```python
from build123d import *

# Parameters (mm, degrees)
F0_R     = 12.7
F1_DEPTH = 60.325
F2_W     = 51.3197111964
F2_H     = 22.6086642011
F3_DEPTH = 55.88
F4_DEPTH = 19.05
F5_DEPTH = 19.05
F6_R     = 6.35
F7_DEPTH = 22.353


with BuildPart() as f1:
    # F0 (on Front) → F1 (new body)
    with BuildSketch(Plane.XZ):
        with BuildLine():
            ThreePointArc((-47.1229317725, 0), (-49.3023607466, 0.8214167326), (-50.3974654162, 2.876990099))
            ThreePointArc((-50.3974654162, 2.876990099), (-89.3551798917, 14.7530576713), (-72.5635393124, -22.352))
            Line((-72.5635393124, -22.352), (19.2828606876, -22.352))
            Line((19.2828606876, -22.352), (13.2884606876, 0))
            Line((13.2884606876, 0), (-47.1229317725, 0))
        make_face()
        with Locations((-72.5635393124, 0)):
            Circle(F0_R, mode=Mode.SUBTRACT)
        Polygon((13.2884606876, 0), (19.2828606876, -22.352), (44.6828606876, -22.352), (44.6828606876, 0), align=None)
        with BuildLine():
            Line((44.6828606876, 0), (44.6828606876, -22.352))
            Line((44.6828606876, -22.352), (121.6448606876, -22.352))
            Line((121.6448606876, -22.352), (121.6448606876, -7.874))
            ThreePointArc((121.6448606876, -7.874), (119.3386194827, -2.3062412049), (113.7708606876, 0))
            Line((113.7708606876, 0), (80.8270606876, 0))
            Line((80.8270606876, 0), (44.6828606876, 0))
        make_face()
    extrude(amount=-F1_DEPTH)

    # F2 (on Top) → F3 (cut, symmetric)
    with BuildSketch(Plane.XY):
        with Locations((-69.2556837142, 30.3035321005)):
            Rectangle(F2_W, F2_H)
    extrude(amount=F3_DEPTH, both=True, mode=Mode.SUBTRACT)

    # F0 (on Front) → F4 (cut)
    with BuildSketch(Plane.XZ):
        Polygon((13.2884606876, 0), (19.2828606876, -22.352), (44.6828606876, -22.352), (44.6828606876, 0), align=None)
    extrude(amount=-F4_DEPTH, mode=Mode.SUBTRACT)

    # F0 (on Front) → F5 (join)
    with BuildSketch(Plane.XZ):
        with BuildLine():
            ThreePointArc((58.4750606876, 34.798), (54.9008760492, 16.0823576341), (44.6828606876, 0))
            Line((44.6828606876, 0), (80.8270606876, 0))
            ThreePointArc((80.8270606876, 0), (78.4921940962, 0.9671334085), (77.5250606876, 3.302))
            Line((77.5250606876, 3.302), (77.5250606876, 29.718))
            ThreePointArc((77.5250606876, 29.718), (76.0371631361, 33.3101024484), (72.4450606876, 34.798))
            Line((72.4450606876, 34.798), (58.4750606876, 34.798))
        make_face()
    extrude(amount=-F5_DEPTH)

    # F6 (on Top) → F7 (cut, through all)
    with BuildSketch(Plane.XY):
        with Locations((82.7828606876, 37.973)):
            Circle(F6_R)
    extrude(amount=-F7_DEPTH, mode=Mode.SUBTRACT)


solid = f1.part
```
Geometry check sheet. Reference: the model listing, model coordinates, mm. A direction names the side the tool comes from. Coordinates: 2 decimals unless noted, no trailing zeros. Order: outer loops, then holes, each group sorted by start corner. A loop starts at its lowest first (then second) coordinate and runs counter-clockwise, first axis right, second up.
Item 1: Section check B-B (x = 87). Enter the section's corners in (y, z) (3 decimals).
Item 2: Scan lines: line 1 along Y through (x, z) = (-49.5, -13.5) (3 decimals); line 2 along Y through (x, z) = (24.5, -9) (3 decimals); line 3 along Z through (x, y) = (1, 27.5). Record each from-to range of solid material in increasing order.
Item 3: Depth check by flat-ended pin: pin 1 (15 mm diameter, centred on y = 11, z = 21, fed in from +X); pin 2 (1.5 mm diameter, centred on x = -52, y = 53, fed in from +Z); pin 3 (11 mm diameter, centred on y = 33, z = -15, fed in from -X). Enter the tip coordinate at first touch or a pass-through.
Item 4: Section check D-D (z = 6). Enter the section's corners in (x, y) (3 decimals), plus the area to 3 significant figures.
Item 5: Tool access check on faces 5 (the flat face through (-64, 18.999, -10)), 6 (the flat face through (34, 36, 0)), 7 (the cylindrical face through (55, 9.39, 16.33)), 8 (the flat face through (16.244, 9.392, -11.02)), 9 (the flat face through (67, 19.05, 18)). Record the directions out of +Z, -Z, +X, -X, +Y, -Y that give a thin tool (end or side, any length) a straight path to the whole face; none if there is none.
Item 6: Section check A-A (z = -10). Enter the section's corners in (x, y) (3 decimals).
Item 7: Mould release check, pull along X, two halves, no side actions. Record for faces 1 (the flat face through (-64, 41.608, -10)), 2 (the cylindrical face through (-60.45, 50.84, 3.81)), 3 (the flat face through (77.525, 9, 16)), 4 (the flat face through (44.683, 9, -11)): released by +X, released by -X, zero draft, split by the parting line, or undercut.
Item 8: Section check C-C (y = 52.5). Enter the section's corners in (x, z), plus the area to 3 significant figures.
Check sheet entries:
1. outline: (0, -22.352) - (33.226, -22.352) - (33.226, 0) - (0, 0) - close; (42.72, -22.352) - (60.325, -22.352) - (60.325, 0) - (42.72, 0) - close
2. line 1: y = 0 to 18.999, 41.608 to 60.325
2. line 2: y = 19.05 to 60.325
2. line 3: z = -22.35 to 0
3. pin 1: stops at x = 77.53
3. pin 2: stops at z = 10.35
3. pin 3: stops at x = -43.6
4. outline: (-94.095, 0) - (-83.757, 0) - (-83.757, 18.999) - (-94.095, 18.999) - close; (-94.095, 41.608) - (-83.757, 41.608) - (-83.757, 60.325) - (-94.095, 60.325) - close; (-61.37, 0) - (-51.032, 0) - (-51.032, 18.999) - (-61.37, 18.999) - close; (-61.37, 41.608) - (-51.032, 41.608) - (-51.032, 60.325) - (-61.37, 60.325) - close; (49.522, 0) - (77.525, 0) - (77.525, 19.05) - (49.522, 19.05) - close
4. area: 1,310 mm2
5. face 5: +Z, -Z, -X
5. face 6: +Z, +Y
5. face 7: +Z, +Y, -Y
5. face 8: +Z, -Y
5. face 9: +Z, +X, -X, +Y
6. outline: (-92.554, 0) - (-80.392, 0) - (-80.392, 18.999) - (-92.554, 18.999) - close; (-92.554, 41.608) - (-80.392, 41.608) - (-80.392, 60.325) - (-92.554, 60.325) - close; (-64.735, 0) - (15.97, 0) - (15.97, 19.05) - (44.683, 19.05) - (44.683, 0) - (121.645, 0) - (121.645, 60.325) - (-64.735, 60.325) - (-64.735, 41.608) - (-43.596, 41.608) - (-43.596, 18.999) - (-64.735, 18.999) - close; hole circle Ø12.7 at (82.783, 37.973)
7. face 1: zero draft
7. face 2: undercut
7. face 3: released by +X
7. face 4: undercut
8. outline: (-72.56, -22.35) - (121.64, -22.35) - (121.64, -7.87) arc R7.87 ccw to (113.77, 0) - (-47.12, 0) arc R3.3 cw to (-50.4, 2.88) arc R22.35 ccw (long way) to start; hole circle Ø25.4 at (-72.56, 0)
8. area: 5,000 mm2
